Could you check a few things on this model? Use its own coordinates, in mm. Face numbers are marked on the shaded views. A direction names the side the tool comes from. Give positions to 0.01 mm unless a question says otherwise; leave off trailing zeros. Order: outer loops, then holes, each group sorted by start corner. A loop starts at its lowest first (then second) coordinate and runs counter-clockwise, first axis right, second up. Notation, with made-up numbers: (2.5, 86) -> (47.5, 86) arc R15 ccw to (47.5, 104) -> close; hole circle Ø2 at (67, -24). An arc over 180 degrees is marked (long way). Write each question's results on one line, items separated by ' | '.
```python
from build123d import *

# Parameters (mm, degrees)
SKETCH1_R                 = 17.37527472527474
BOSS_EXTRUDE1_DEPTH       = 2.54
BOSS_EXTRUDE2_START       = -5.175
BOSS_EXTRUDE2_OUTLINE_R   = 17.375274725
BOSS_EXTRUDE2_OUTLINE_R_2 = 1
BOSS_EXTRUDE2_OUTLINE_R_3 = 4.25
BOSS_EXTRUDE2_DEPTH       = 2.635
SKETCH2_R                 = 9.525
BOSS_EXTRUDE4_DEPTH       = 19.05
CHAMFER1_SIZE             = 12.7
CHAMFER1_SIZE2            = 2.23935265499751


# Read off the part's stored shape, not the designer's step: Boss-Extrude2
with BuildPart() as part:
    # Sketch1 → Boss-Extrude1 (new body)
    with BuildSketch(Plane(origin=(0, 325.36739999999986, 0), x_dir=(1, 0, 0), z_dir=(0, 1, 0))):
        with Locations(Location((0, 3.66e-14, 0), (0, 0, 270))):
            Circle(SKETCH1_R)
        with BuildLine():
            Line((-8.83112529829345, -3.568872506245661), (-14.736178288860136, -1.88495193133948))
            ThreePointArc((-14.736178288860136, -1.8849519313394787), (-16.73655161171898, 0.9233006813963234), (-14.43941301600355, 3.49447365103826))
            Line((-14.43941301600355, 3.4944736510382595), (-8.384964425073763, 4.51862773308911))
            ThreePointArc((-8.384964425073935, 4.518627733089421), (-7.974035718754682, 5.209642920203345), (-7.506296902423261, 5.863542599203262))
            Line((-7.506296902423427, 5.863542599203276), (-9.000505401882572, 11.81942878717986))
            ThreePointArc((-9.000505401882574, 11.81942878717986), (-7.5686739604387565, 14.955929208196205), (-4.1934035533472525, 14.25213531311389))
            Line((-4.193403553347251, 14.25213531311389), (-0.2792358054370207, 9.520906068487482))
            ThreePointArc((-0.27923580543699295, 9.520906068487529), (0.5246652541642909, 9.510538963227763), (1.3248283958705547, 9.432415105448642))
            Line((1.3248283958705054, 9.432415105448754), (5.7356728869774125, 13.70438071851937))
            ThreePointArc((5.7356728869774125, 13.70438071851937), (9.16787765128006, 14.03262852679995), (10.246009462656167, 10.75766166207572))
            Line((10.246009462656167, 10.75766166207572), (8.1057286196369, 5.0022783353981914))
            ThreePointArc((8.105728619637244, 5.002278335398186), (8.498700972919012, 4.300896043024725), (8.831125298293639, 3.5688725062459628))
            Line((8.831125298293461, 3.5688725062457136), (14.736178288860124, 1.884951931339582))
            ThreePointArc((14.736178288860126, 1.8849519313395824), (16.736551611718987, -0.9233006813962088), (14.43941301600357, -3.494473651038158))
            Line((14.43941301600357, -3.4944736510381578), (8.384964425073758, -4.518627733089059))
            ThreePointArc((8.384964425073925, -4.518627733089367), (7.974035718754691, -5.20964292020326), (7.506296902423297, -5.863542599203144))
            Line((7.5062969024234505, -5.863542599203156), (9.000505401882656, -11.8194287871798))
            ThreePointArc((9.000505401882656, -11.8194287871798), (7.568673960438859, -14.955929208196153), (4.193403553347351, -14.252135313113861))
            Line((4.193403553347352, -14.252135313113861), (0.2792358054370711, -9.520906068487413))
            ThreePointArc((0.2792358054370489, -9.520906068487452), (-0.5246652541641907, -9.510538963227694), (-1.3248283958704137, -9.432415105448587))
            Line((-1.3248283958703642, -9.432415105448698), (-5.735672886977412, -13.70438071851937))
            ThreePointArc((-5.7356728869774125, -13.70438071851937), (-9.167877651280058, -14.032628526799948), (-10.246009462656165, -10.75766166207572))
            Line((-10.246009462656165, -10.75766166207572), (-8.105728619636901, -5.002278335398116))
            ThreePointArc((-8.105728619637246, -5.002278335398109), (-8.498700972919007, -4.300896043024661), (-8.83112529829363, -3.56887250624591))
        make_face(mode=Mode.SUBTRACT)
    extrude(amount=-BOSS_EXTRUDE1_DEPTH)

    # Boss-Extrude2 outline → Boss-Extrude2 (add)
    with BuildSketch(Plane(origin=(0, 325.36739999999986, 0), x_dir=(1, 0, 0), z_dir=(0, 1, 0)).offset(BOSS_EXTRUDE2_START)):
        Circle(BOSS_EXTRUDE2_OUTLINE_R)
        with Locations((-4.10208104, -6.278768282)):
            Circle(BOSS_EXTRUDE2_OUTLINE_R_2, mode=Mode.SUBTRACT)
        with Locations((3.386532317, -6.69189053)):
            Circle(BOSS_EXTRUDE2_OUTLINE_R_2, mode=Mode.SUBTRACT)
        with Locations((7.488613357, -0.413122247)):
            Circle(BOSS_EXTRUDE2_OUTLINE_R_2, mode=Mode.SUBTRACT)
        with Locations((-7.488613357, 0.413122247)):
            Circle(BOSS_EXTRUDE2_OUTLINE_R_2, mode=Mode.SUBTRACT)
        with Locations((-3.386532317, 6.69189053)):
            Circle(BOSS_EXTRUDE2_OUTLINE_R_2, mode=Mode.SUBTRACT)
        Circle(BOSS_EXTRUDE2_OUTLINE_R_3, mode=Mode.SUBTRACT)
        with Locations((4.10208104, 6.278768282)):
            Circle(BOSS_EXTRUDE2_OUTLINE_R_2, mode=Mode.SUBTRACT)
    extrude(amount=BOSS_EXTRUDE2_DEPTH)

    # Sketch2 → Boss-Extrude4 (add)
    with BuildSketch(Plane.XZ.offset(-320.19239999999985)):
        with Locations(Location((0, 0, 0), (0, 0, 90))):
            Circle(SKETCH2_R)
    extrude(amount=BOSS_EXTRUDE4_DEPTH)

    # Chamfer1
    chamfer1_edges = [part.edges().sort_by_distance(p)[0] for p in [
        (-1.75e-15, 301.14239999999984, -9.525),
    ]]
    chamfer1_side = [part.faces().sort_by_distance(p)[0] for p in [
        (-1.75e-15, 310.6673999999999, -9.525),
    ]]
    chamfer(chamfer1_edges, length=CHAMFER1_SIZE, length2=CHAMFER1_SIZE2, reference=chamfer1_side[0])


solid = part.part
```
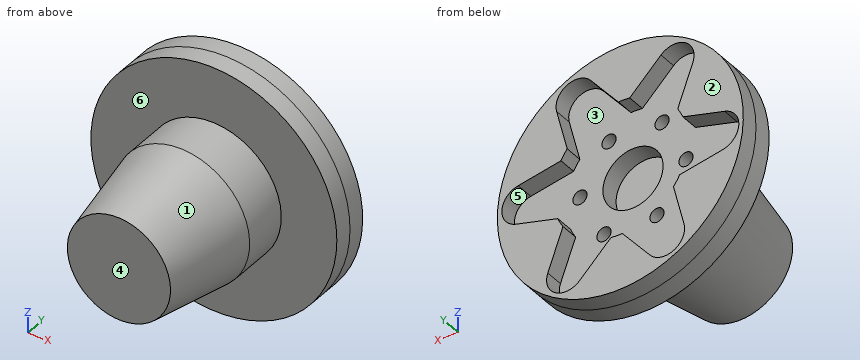
Q1. I need wall thicknesses on line 1 along X through (y, z) = (324, 10); line 2 along Z through (x, y) = (4, 309); line 3 along Y through (x, z) = (-8, -9). Which ranges of each line are inside material? Lowest first, please.
Here are the results:
line 1: x = -14.21 to -9.96, -1.91 to 0.68, 8.54 to 14.21 | line 2: z = -7.69 to 7.69 | line 3: y = 320.19 to 322.83
Q2. Suppose I cut it at A-A on y = 319.5. Please give me the cut outline in (x, z) (3 decimals).
Here are the results:
outline: circle Ø19.05 at (0, 0)
Q3. For the marked faces 4, 5 and 6, which set-ups out of +Z, -Z, +X, -X, +Y, -Y let a thin tool reach every point of the face, with its end or its side?
Here are the results:
face 4: +Z, -Z, +X, -X, -Y | face 5: +Y | face 6: -Y
Q4. I'm going to push flat-ended pins straight in: pin 1 Ø1.5 at (x, z) = (-8.5, 12.5) entering from -Y; pin 2 Ø9 at (x, z) = (4.5, -5.5) entering from +Y; pin 3 Ø3 at (y, z) = (318, -7) entering from +X; pin 4 Ø1 at (x, z) = (-4.5, 6.5) entering from +Y. Where does each tip first touch, or does it pass through?
Here are the results:
pin 1: stops at y = 320.19 | pin 2: stops at y = 325.37 | pin 3: stops at x = 7.78 | pin 4: stops at y = 320.19
Q5. Thinking about a two-plate mould opening in X: for the marked faces 1, 2 and 3, which applies, +X half, -X half, draft (parallel to the pull), parting line (faces both ways), or undercut?
Here are the results:
face 1: parting line | face 2: draft | face 3: undercut
Q6. Suppose I cut it at C-C on y = 312. Please give me the cut outline in (x, z), and give its area (3 significant figures).
Here are the results:
outline: circle Ø18.4 at (0, 0) | area: 266 mm²
Q7. Suppose I cut it at B-B on z = 13. Please give me the cut outline in (x, y).
Here are the results:
outline: (-11.53, 320.19) -> (11.53, 320.19) -> (11.53, 325.37) -> (9.04, 325.37) -> (9.04, 322.83) -> (3.16, 322.83) -> (3.16, 325.37) -> (-5.01, 325.37) -> (-5.01, 322.83) -> (-10.1, 322.83) -> (-10.1, 325.37) -> (-11.53, 325.37) -> close
